Source: CAD feature listing. Evaluate the final solid. Frame: model axes, mm. Face numbers are marked on the shaded views. A direction names the side the tool comes from. Round coordinates to 2 decimals unless told otherwise and drop trailing zeros. Write each loop counter-clockwise with the first axis right and the second up, starting at its lowest first coordinate (ties: lowest second). Pieces come first, ordered by that corner, then holes.
from build123d import *

# Parameters (mm, degrees)
BOSS_EXTRUDE_DEPTH      = 50.8
BOSS_EXTRUDE_DEPTH_BACK = 0.01
SKETCH1_R               = 17.5
SKETCH2_R               = 4.5
CUT_EXTRUDE1_DEPTH      = 64.101758025
SKETCH3_R               = 11.5
CUT_EXTRUDE3_DEPTH      = 8


# Read off the part's stored shape, not the designer's step: Draft3
with BuildPart() as part:
    # Sketch1 → Boss-Extrude (new, two sides: drawn at the far end of the back side and taken through both)
    with BuildSketch(Plane.XY.offset(-BOSS_EXTRUDE_DEPTH_BACK)):
        Circle(SKETCH1_R)
    extrude(amount=BOSS_EXTRUDE_DEPTH + BOSS_EXTRUDE_DEPTH_BACK)

    # Draft3 outline → Draft3 (revolve)
    with BuildSketch(Plane.XZ):
        Polygon((26.45917389, -0.01), (17.5, 50.8), (17.5, -0.01), align=None)
    revolve(axis=Axis((0, 0, 0), (0, 0, 1)))

    # Sketch2 → Cut-Extrude1 (cut, through all)
    with BuildSketch(Plane(origin=(0, 0, -0.01), x_dir=(-1, 0, 0), z_dir=(0, 0, -1))):
        Circle(SKETCH2_R)
    extrude(amount=-CUT_EXTRUDE1_DEPTH, mode=Mode.SUBTRACT)

    # Sketch3 → Cut-Extrude3 (cut)
    with BuildSketch(Plane(origin=(0, 0, -0.01), x_dir=(-1, 0, 0), z_dir=(0, 0, -1))):
        Circle(SKETCH3_R)
    extrude(amount=-CUT_EXTRUDE3_DEPTH, mode=Mode.SUBTRACT)


solid = part.part
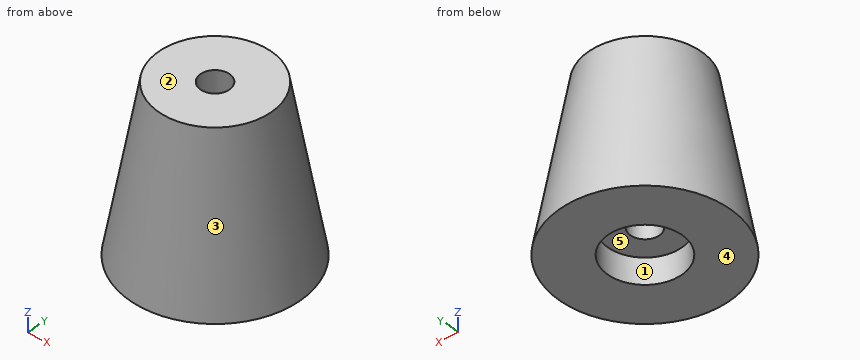
1) Section query D-D on z = 12.5. Return the cut outline in (x, y).
Taken from the geometry:
outline: circle Ø48.51 at (0, 0); hole circle Ø9 at (0, 0)
2) Reachability of the marked faces 4 and 5 from +Z, -Z, +X, -X, +Y, -Y: full face, straight path, thin tool, end or side. Return the list, or none.
Taken from the geometry:
face 4: -Z, +X, -X, +Y, -Y
face 5: -Z
3) Section query C-C on z = 46. Return the cut outline in (x, y), then the cut area to 3 significant figures.
Taken from the geometry:
outline: circle Ø36.69 at (0, 0); hole circle Ø9 at (0, 0)
area: 994 mm2
4) Pull-direction query (X, two-part tool) for the marked faces 1, 2 and 3; classes: released by +X, released by -X, zero draft, split by the parting line, or undercut.
Taken from the geometry:
face 1: undercut
face 2: zero draft
face 3: split by the parting line
5) Material intervals for line 1 (Y direction, x = 0, z = 5.25); line 2 (X direction, y = 3, z = 31); line 3 (Y direction, x = 0, z = 5), sorted ascending.
Taken from the geometry:
line 1: y = -25.53 to -11.5, 11.5 to 25.53
line 2: x = -20.78 to -3.35, 3.35 to 20.78
line 3: y = -25.58 to -11.5, 11.5 to 25.58
6) Section query A-A on y = 0. Return the cut outline in (x, z).
Taken from the geometry:
outline: (-26.46, -0.01) - (-11.5, -0.01) - (-11.5, 7.99) - (-4.5, 7.99) - (-4.5, 50.8) - (-17.5, 50.8) - close; (4.5, 7.99) - (11.5, 7.99) - (11.5, -0.01) - (26.46, -0.01) - (17.5, 50.8) - (4.5, 50.8) - close
7) Contact query for flat-ended pins moving along their axis: P1, Ø12, axis at x = 14.5, z = 35, coming from the +Y side; P2, Ø8, axis at x = 19, y = -9, coming from the +Z side; P3, Ø6, axis at y = -7, z = 34.5, coming from the -X side; P4, Ø8, axis at x = 0, y = 0, coming from the -Z side. Output: stop coordinate, or through.
Taken from the geometry:
P1: stops at y = 18.65
P2: stops at z = 50.8
P3: stops at x = -20.17
P4: passes through
